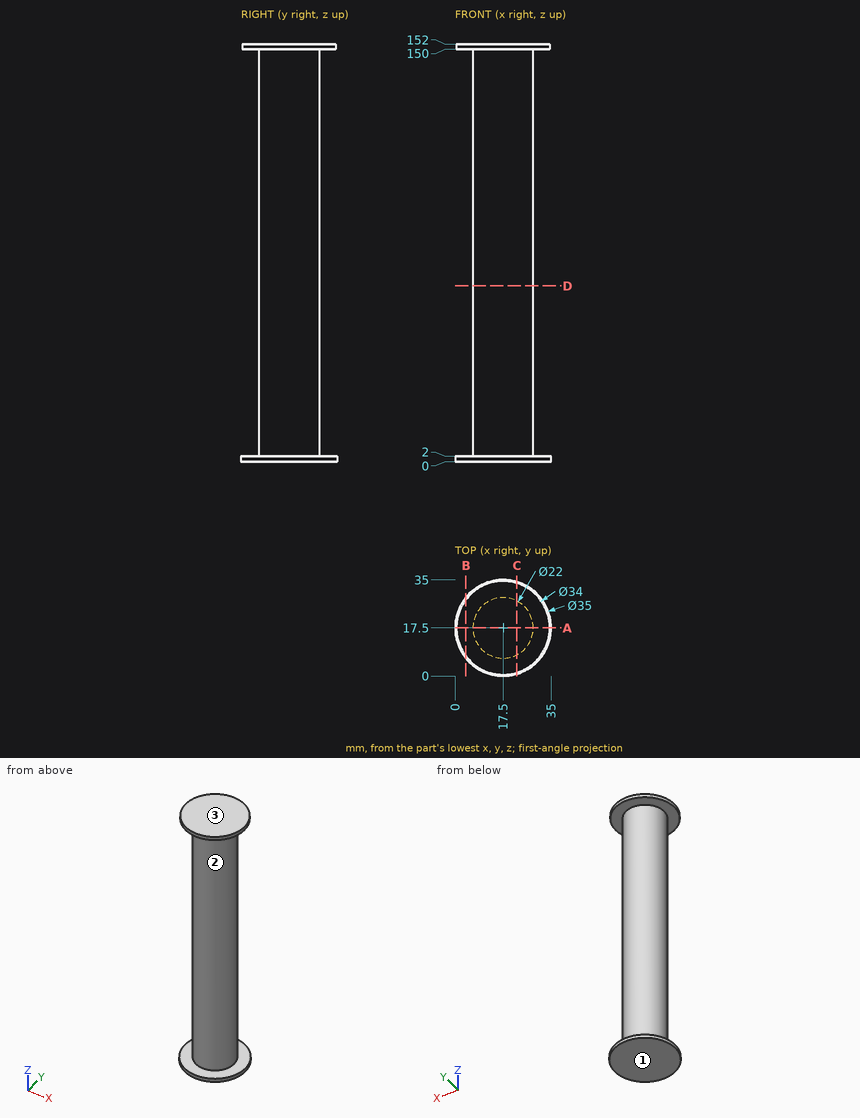
Print and shaded views of the part. All mm, measured from the part's lowest x, y and z. Round coordinates to 2 decimals unless told otherwise and drop trailing zeros. Write each loop counter-clockwise with the first axis right and the second up, starting at its lowest first coordinate (ties: lowest second). Pieces come first, ordered by that corner, then holes. Notation, with made-up numbers: (20.5, 45) - (45.5, 45) arc R16 cw to (45.5, 73) - close; hole circle Ø7 at (83, 58.25). An arc over 180 degrees is marked (long way). Write each question's results on one line, items separated by ' | '. Start each with the question number.
Item 1: Saw through at D-D (z = 64). Write the cut outline in (x, y), and give its area (3 significant figures).
Item 2: Saw through at A-A (y = 17.5). Write the cut outline in (x, z), and give its area (3 significant figures).
Item 3: Wall check: L1, parallel to Z at x = 29, y = 23.5; L2, parallel to X at y = 12, z = 134; L3, parallel to Y at x = 11.5, z = 51.5. Give the ranges that are in metal, low to high. Write a range as [from, to].
Item 4: Saw through at C-C (x = 22.5). Write the cut outline in (y, z), and give its area (3 significant figures).
Item 5: Drop flat-ended pins along their axis: P1, Ø4, axis at y = 11, z = 113.5, coming from the +X side; P2, Ø1.5, axis at y = 16.5, z = 51.5, coming from the -X side; P3, Ø12, axis at x = 31, z = 115, coming from the -Y side. Give the stop position or say it passes through.
Item 6: Saw through at B-B (x = 4). Write the cut outline in (y, z), and give its area (3 significant figures).
Item 7: Mould opens along Z. For the marked faces 1, 2 and 3 say: pulls with the +Z half, pulls with the -Z half, needs draft (parallel to the pull), parting line crosses it, or undercut.
Results are:
1) outline: circle Ø22 at (17.5, 17.5) | area: 380 mm²
2) outline: (0, 0) - (35, 0) - (35, 2) - (28.5, 2) - (28.5, 150) - (34.5, 150) - (34.5, 152) - (0.5, 152) - (0.5, 150) - (6.5, 150) - (6.5, 2) - (0, 2) - close | area: 3,390 mm²
3) L1: z = [0, 2], [150, 152] | L2: x = [7.97, 27.03] | L3: y = [8.28, 26.72]
4) outline: (0.73, 0) - (34.27, 0) - (34.27, 2) - (27.3, 2) - (27.3, 150) - (33.75, 150) - (33.75, 152) - (1.25, 152) - (1.25, 150) - (7.7, 150) - (7.7, 2) - (0.73, 2) - close | area: 3,030 mm²
5) P1: stops at x = 27.54 | P2: stops at x = 6.5 | P3: stops at y = 9.45
6) outline: (6.36, 0) - (28.64, 0) - (28.64, 2) - (6.36, 2) - close; (7.17, 150) - (27.83, 150) - (27.83, 152) - (7.17, 152) - close | area: 85.9 mm²
7) face 1: pulls with the -Z half | face 2: undercut | face 3: pulls with the +Z half
